Build history of the part. All positions in model axes, mm. Face numbers are marked on the shaded views. A direction names the side the tool comes from. Round coordinates to 2 decimals unless told otherwise and drop trailing zeros. Write each loop counter-clockwise with the first axis right and the second up, starting at its lowest first coordinate (ties: lowest second). Pieces come first, ordered by that corner, then holes. Notation, with made-up numbers: M -33.75,-16.75 L 8.25,-16.75 A34 cw 8.25,14.25 Z; hole C 38.25,53 d2. An arc over 180 degrees is marked long. One line per item, written item: value. Start each with the question number.
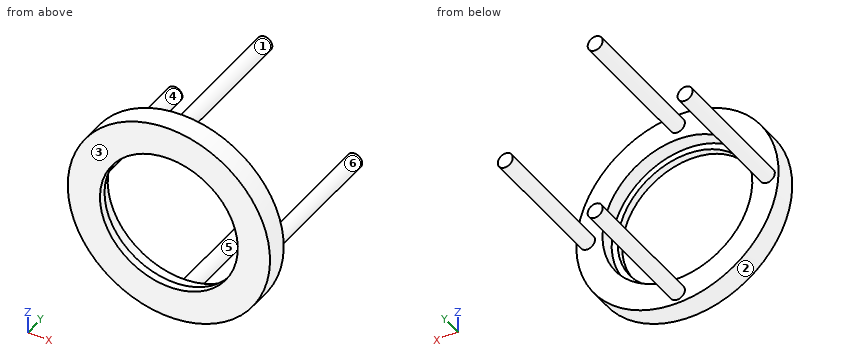
```python
from build123d import *

# Parameters (mm, degrees)
SKETCH1_R           = 33.75
BOSS_EXTRUDE1_DEPTH = 7.5
SKETCH2_R           = 2.5
BOSS_EXTRUDE2_DEPTH = 45
SKETCH3_R           = 25
CUT_EXTRUDE1_DEPTH  = 5
SKETCH4_R           = 23
CUT_EXTRUDE2_DEPTH  = 70.123982813


with BuildPart() as part:
    # Sketch1 → Boss-Extrude1 (new body)
    with BuildSketch(Plane(origin=(0, 0, 0), x_dir=(1, 0, 0), z_dir=(0, 1, 0))):
        with Locations(Location((0, 0, 0), (0, 0, 270))):
            Circle(SKETCH1_R)
    extrude(amount=BOSS_EXTRUDE1_DEPTH)

    # Sketch2 → Boss-Extrude2 (add)
    with BuildSketch(Plane(origin=(0, 7.5, 0), x_dir=(1, 0, 0), z_dir=(0, 1, 0))):
        with Locations(Location((-30, 0, 0), (0, 0, 90))):
            Circle(SKETCH2_R)
        with Locations(Location((30, 0, 0), (0, 0, 90))):
            Circle(SKETCH2_R)
        with Locations(Location((0, -30, 0), (0, 0, 90))):
            Circle(SKETCH2_R)
        with Locations(Location((0, 30, 0), (0, 0, 90))):
            Circle(SKETCH2_R)
    extrude(amount=BOSS_EXTRUDE2_DEPTH)

    # Sketch3 → Cut-Extrude1 (cut)
    with BuildSketch(Plane(origin=(0, 7.5, 0), x_dir=(1, 0, 0), z_dir=(0, 1, 0))):
        with Locations(Location((0, 0, 0), (0, 0, 270))):
            Circle(SKETCH3_R)
    extrude(amount=-CUT_EXTRUDE1_DEPTH, mode=Mode.SUBTRACT)

    # Sketch4 → Cut-Extrude2 (cut, through all)
    with BuildSketch(Plane(origin=(0, 2.5, 0), x_dir=(1, 0, 0), z_dir=(0, 1, 0))):
        with Locations(Location((0, 0, 0), (0, 0, 270))):
            Circle(SKETCH4_R)
    extrude(amount=-CUT_EXTRUDE2_DEPTH, mode=Mode.SUBTRACT)


solid = part.part
```
Item 1: Cut at C-C, the plane y = 21. Write the cut outline in (x, z), plus the area to 3 significant figures.
Item 2: Drop flat-ended pins along their axis: pin 1 (2 mm diameter, centred on x = 9.5, y = 10, fed in from +Z); pin 2 (4 mm diameter, centred on y = 35, z = 0.5, fed in from +X); pin 3 (6 mm diameter, centred on x = -25, y = 21.5, fed in from -Z). Give the stop position or say it passes through.
Item 3: Cut at D-D, the plane x = -11. Write the cut outline in (y, z), plus the area to 3 significant figures.
Item 4: Cut at B-B, the plane z = 0. Write the cut outline in (x, y), plus the area to 3 significant figures.
Item 5: Cut at A-A, the plane x = 0. Write the cut outline in (y, z), plus the area to 3 significant figures.
Item 6: Two-plate mould, pull along X, no slides. Class the marked faces 3, 4, 5 and 6: pulls with the +X half, pulls with the -X half, needs draft (parallel to the pull), parting line crosses it, or undercut.
Item 7: Which spindle directions (+Z, -Z, +X, -X, +Y, -Y) get a long thin tool onto all of the face, cutting with end or side? Do the marked faces 1 and 2. Say none if no direction does.
Item 8: Drill centre lines: line 1 (X direction, y = 5, z = 0); line 2 (Y direction, x = -9, z = 24.5); line 3 (X direction, y = 0.55, z = 0). Where is each one in solid material? Low to high.
Computed values:
1. outline: C -30,0 d5; C 0,-30 d5; C 0,30 d5; C 30,0 d5
1. area: 78.5 mm2
2. pin 1: passes through
2. pin 2: stops at x = 32.5
2. pin 3: stops at z = -1.5
3. outline: M 0,-31.91 L 7.5,-31.91 L 7.5,-22.45 L 2.5,-22.45 L 2.5,-20.2 L 0,-20.2 Z; M 0,20.2 L 2.5,20.2 L 2.5,22.45 L 7.5,22.45 L 7.5,31.91 L 0,31.91 Z
3. area: 153 mm2
4. outline: M -33.75,0 L -23,0 L -23,2.5 L -25,2.5 L -25,7.5 L -27.5,7.5 L -27.5,52.5 L -32.5,52.5 L -32.5,7.5 L -33.75,7.5 Z; M 23,0 L 33.75,0 L 33.75,7.5 L 32.5,7.5 L 32.5,52.5 L 27.5,52.5 L 27.5,7.5 L 25,7.5 L 25,2.5 L 23,2.5 Z
4. area: 591 mm2
5. outline: M 0,-33.75 L 7.5,-33.75 L 7.5,-32.5 L 52.5,-32.5 L 52.5,-27.5 L 7.5,-27.5 L 7.5,-25 L 2.5,-25 L 2.5,-23 L 0,-23 Z; M 0,23 L 2.5,23 L 2.5,25 L 7.5,25 L 7.5,27.5 L 52.5,27.5 L 52.5,32.5 L 7.5,32.5 L 7.5,33.75 L 0,33.75 Z
5. area: 591 mm2
6. face 3: needs draft
6. face 4: undercut
6. face 5: parting line crosses it
6. face 6: undercut
7. face 1: +Y
7. face 2: +Y, -Y
8. line 1: x = -33.75 to -25, 25 to 33.75
8. line 2: y = 0 to 7.5
8. line 3: x = -33.75 to -23, 23 to 33.75
